Check sheet for the modelled part. Datum: model origin and axes. Units: mm. Face numbers are marked on the shaded views. Round coordinates to 2 decimals unless told otherwise and drop trailing zeros. Order: outer loops, then holes, each group sorted by start corner. A loop starts at its lowest first (then second) coordinate and runs counter-clockwise, first axis right, second up.
Autodesk Inventor part; units mm, degrees
ref_plane "YZ Plane" through (0, 0, 0) normal (1, 0, 0) x (0, 1, 0)
ref_plane "XZ Plane" through (0, 0, 0) normal (0, 1, 0) x (-1, 0, 0)
ref_plane "XY Plane" through (0, 0, 0) normal (0, 0, 1) x (1, 0, 0)
sketch "スケッチ1" plane through (0, 0, 0) normal (0, 1, 0) x (-1, 0, 0)
  line L0 (0, 0) -> (4, 0)
  line L1 (4, 0) -> (4, -1.5)
  line L2 (4, -1.5) -> (0, -1.5)
  line L3 (0, -1.5) -> (0, 0)
  dimension "d0" = 4
  dimension "d1" = 1.5
extrude "押し出し1" add sketch "スケッチ1" along normal blind 8
sketch "スケッチ2" plane through (-4, 0, 0) normal (0, 0, 1) x (1, 0, 0)
  circle A0 centre (2, 5.933) radius 0.8201
  line L0 (0, 0) -> (0, 8)
  point P0 (4, 0)
  dimension "d4" = 2
extrude "押し出し2" cut sketch "スケッチ2" against normal blind 8
fillet "フィレット1" radius 1 2 edges at (0, 8, -0.75) (-4, 8, -0.75)
properties part number "モーター端子"
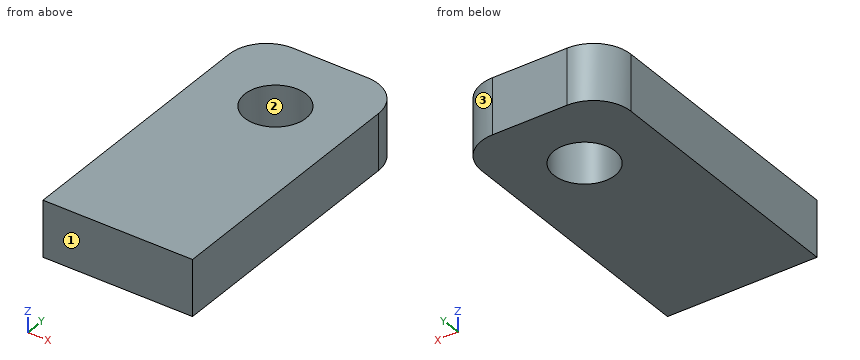
1) Sectioned sample at C-C on z = -1.15. Record the cut outline in (x, y), and give its area (3 significant figures).
2) Draft check along Y on the marked faces 1, 2 and 3. Enter one of: pulls with the +Y half, pulls with the -Y half, needs draft (parallel to the pull), parting line crosses it, or undercut.
3) Sectioned sample at A-A on x = -2. Record the cut outline in (y, z).
4) Sectioned sample at B-B on y = 5.25. Record the cut outline in (x, z), and give its area (3 significant figures).
5) Scan lines: line 1 (Y direction, x = -2, z = -0.9); line 2 (X direction, y = 6, z = -1.05); line 3 (Y direction, x = -1.4, z = -1). Record each from-to range of solid material in increasing order.
Values found:
1. outline: (-4, 0) - (0, 0) - (0, 7) arc R1 ccw to (-1, 8) - (-3, 8) arc R1 ccw to (-4, 7) - close; hole circle Ø1.64 at (-2, 5.93)
1. area: 29.5 mm2
2. face 1: pulls with the -Y half
2. face 2: undercut
2. face 3: pulls with the +Y half
3. outline: (0, -1.5) - (5.11, -1.5) - (5.11, 0) - (0, 0) - close; (6.75, -1.5) - (8, -1.5) - (8, 0) - (6.75, 0) - close
4. outline: (-4, -1.5) - (-2.45, -1.5) - (-2.45, 0) - (-4, 0) - close; (-1.55, -1.5) - (0, -1.5) - (0, 0) - (-1.55, 0) - close
4. area: 4.64 mm2
5. line 1: y = 0 to 5.11, 6.75 to 8
5. line 2: x = -4 to -2.82, -1.18 to 0
5. line 3: y = 0 to 5.37, 6.49 to 8
